from build123d import *

# Parameters (mm, degrees)
F0_W     = 73.7051814795
F0_H     = 58.4876872599
F1_DEPTH = 25.4
F2_T     = -2.54
F3_R     = 5.08
F4_R     = 5.08


with BuildPart() as f1:
    # F0 (on Top) → F1 (new body)
    with BuildSketch(Plane.XY):
        with Locations((36.8525907397, -29.24384363)):
            Rectangle(F0_W, F0_H)
    extrude(amount=F1_DEPTH)

    # F2
    f2_openings = [f1.faces().sort_by_distance(p)[0] for p in [
        (36.852591, -29.243844, 25.4),
    ]]
    offset(amount=F2_T, openings=f2_openings)

    # F3
    f3_edges = [f1.edges().sort_by_distance(p)[0] for p in [
        (0, -58.487687, 12.7),
        (0, 0, 12.7),
        (2.54, -55.947687, 13.97),
        (2.54, -2.54, 13.97),
        (73.705181, 0, 12.7),
        (71.165181, -2.54, 13.97),
        (71.165181, -55.947687, 13.97),
        (73.705181, -58.487687, 12.7),
    ]]
    fillet(f3_edges, radius=F3_R)

    # F4
    f4_edges = [f1.edges().sort_by_distance(p)[0] for p in [
        (71.165181, -29.243844, 2.54),
    ]]
    fillet(f4_edges, radius=F4_R)


solid = f1.part
The listing builds one solid part. Answer for the finished solid, in the listing's coordinates (mm). A direction names the side the tool comes from. Round coordinates to 2 decimals unless told otherwise and drop trailing zeros. Loops run counter-clockwise (first coordinate to the right, second up) from the corner with the lowest first, then second, coordinate; pieces in that order, holes last. Notation, with made-up numbers: M 21,57 L 27,57 A9 ccw 27,65 Z; hole C 10,34 d7. An arc over 180 degrees is marked long. Return JSON: item names as keys, results as strings.
Q1. Which of the six approach directions +Z, -Z, +X, -X, +Y, -Y give full straight-line access (tool end or side, diameter ignored) to faces 4 (the face through (0, -30, 13)), 5 (the face through (69.638, -54.499, 16.634))?
Results list:
{"face 4": "+Z, -Z, -X, +Y, -Y", "face 5": "+Z"}
Q2. Find section A-A, the plane z = 20.5. Determine the outline of the cut face in (x, y), plus the area to 3 significant figures.
Results list:
{"outline": "M 0,-53.41 A5.08 ccw 5.08,-58.49 L 68.63,-58.49 A5.08 ccw 73.71,-53.41 L 73.71,-5.08 A5.08 ccw 68.63,0 L 5.08,0 A5.08 ccw 0,-5.08 Z; hole M 2.54,-50.87 A5.08 ccw 7.62,-55.95 L 66.09,-55.95 A5.08 ccw 71.17,-50.87 L 71.17,-7.62 A5.08 ccw 66.09,-2.54 L 7.62,-2.54 A5.08 ccw 2.54,-7.62 Z", "area": "646 mm2"}
Q3. Find the intervals of material crossed by line 1 along Y through (x, z) = (64.5, 18.25); line 2 along X through (y, z) = (-26, 15); line 3 along Z through (x, y) = (14.5, -50), in increasing order. Write a range as from..to.
Results list:
{"line 1": "y = -58.49..-55.95, -2.54..0", "line 2": "x = 0..2.54, 71.17..73.71", "line 3": "z = 0..2.54"}
Q4. This flat-tipped pin is pushed along its axis until it touches: pin 1 Ø1 at (x, y) = (32.5, -11) entering from +Z. Where does it stop, or does it pass through?
Results list:
{"pin 1": "stops at z = 2.54"}
Q5. The mould has two halves that part along X. Classify faces 1 (the face through (1.449, -1.528, 12.878)), 2 (the face through (3.99, -54.42, 16.39)), 3 (the face through (36, 0, 13)): released by +X, released by -X, zero draft, split by the parting line, or undercut.
Results list:
{"face 1": "released by -X", "face 2": "undercut", "face 3": "zero draft"}
Q6. Find section B-B, the plane x = 32.5. Determine the outline of the cut face in (y, z), plus the area to 3 significant figures.
Results list:
{"outline": "M -58.49,0 L 0,0 L 0,25.4 L -2.54,25.4 L -2.54,7.62 A5.08 cw -7.62,2.54 L -50.87,2.54 A5.08 cw -55.95,7.62 L -55.95,25.4 L -58.49,25.4 Z", "area": "276 mm2"}
Q7. Find section C-C, the plane y = -15. Determine the outline of the cut face in (x, z), plus the area to 3 significant figures.
Results list:
{"outline": "M 0,0 L 73.71,0 L 73.71,25.4 L 71.17,25.4 L 71.17,7.62 A5.08 cw 66.09,2.54 L 7.62,2.54 A5.08 cw 2.54,7.62 L 2.54,25.4 L 0,25.4 Z", "area": "314 mm2"}
